```python
from build123d import *
from build123d import SkipClean  # not in build123d's __all__

# Parameters (mm, degrees)
F1_DEPTH = 9
F2_DEPTH = 13
F4_DEPTH = 2.5
F6_DEPTH = 6
F7_R     = 0.5
F8_DEPTH = 10
F9_DEPTH = 2


with BuildPart() as f1:
    # F0 (on Top) → F1 (new body)
    with BuildSketch(Plane.XY):
        with BuildLine():
            ThreePointArc((9.210061901, 13.0833772314), (-14.201425816, -7.3701767138), (16, 0))
            ThreePointArc((16, 0), (15.9921779437, 0.5002445588), (15.9687194227, 1))
            ThreePointArc((15.9687194227, 1), (13.964052369, 7.8105852172), (9.210061901, 13.0833772314))
        make_face()
        with BuildLine():
            Line((10.5963823009, 7.5310478775), (11.473873387, 8.0218594789))
            ThreePointArc((11.473873387, 8.0218594789), (12.2185458229, 6.834262065), (12.8407258, 5.5781503143))
            Line((12.8407258, 5.5781503143), (11.9632347139, 5.0873387129))
            ThreePointArc((11.9632347139, 5.0873387129), (11.1687805133, -6.6526943298), (1.2238876286, -12.9422601995))
            Line((1.2238876286, -12.9422601995), (1.2101974008, -13.9475955724))
            ThreePointArc((1.2101974008, -13.9475955724), (-0.190628347, -13.9987021125), (-1.5895430217, -13.909469903))
            Line((-1.5895430217, -13.909469903), (-1.5758527939, -12.9041345301))
            ThreePointArc((-1.5758527939, -12.9041345301), (-11.3457925498, -6.346100489), (-11.8202699295, 5.4112123221))
            Line((-11.8202699295, 5.4112123221), (-12.6840707878, 5.9257360935))
            ThreePointArc((-12.6840707878, 5.9257360935), (-12.0279174759, 7.1644400474), (-11.2511827783, 8.3313195887))
            Line((-11.2511827783, 8.3313195887), (-10.38738192, 7.8167958172))
            ThreePointArc((-10.38738192, 7.8167958172), (0.1770120365, 12.9987948187), (10.5963823009, 7.5310478775))
        make_face(mode=Mode.SUBTRACT)
        with BuildLine():
            ThreePointArc((9.210061901, 13.0833772314), (13.964052369, 7.8105852172), (15.9687194227, 1))
            Line((15.9687194227, 1), (18.9687194227, 1))
            Line((18.9687194227, 1), (18.9687194227, 16))
            Line((18.9687194227, 16), (12.4687194227, 16))
            Line((12.4687194227, 16), (9.210061901, 13.0833772314))
        make_face()
    extrude(amount=F1_DEPTH)

    # F0 (on Top) → F2 (join)
    with BuildSketch(Plane.XY):
        with BuildLine():
            ThreePointArc((9.210061901, 13.0833772314), (13.964052369, 7.8105852172), (15.9687194227, 1))
            Line((15.9687194227, 1), (18.9687194227, 1))
            Line((18.9687194227, 1), (18.9687194227, 16))
            Line((18.9687194227, 16), (12.4687194227, 16))
            Line((12.4687194227, 16), (9.210061901, 13.0833772314))
        make_face()
    extrude(amount=F2_DEPTH)

    # F3 (on face) → F4 (join)
    with BuildSketch(Plane.YZ.offset(18.9687194227)):
        with BuildLine():
            Line((3.85, 8.35), (3.85, 0))
            Line((3.85, 0), (13.15, 0))
            Line((13.15, 0), (13.15, 8.35))
            ThreePointArc((13.15, 8.35), (11.7880465325, 11.6380465325), (8.5, 13))
            ThreePointArc((8.5, 13), (5.2119534675, 11.6380465325), (3.85, 8.35))
        make_face()
    extrude(amount=F4_DEPTH)

    # F5 (on face) → F6 (join)
    with BuildSketch(Plane.YZ.offset(21.4687194227)):
        with BuildLine():
            Line((0.5, 23), (0.5, 0))
            Line((0.5, 0), (3.85, 0))
            Line((3.85, 0), (3.85, 8.35))
            ThreePointArc((3.85, 8.35), (8.5, 13), (13.15, 8.35))
            Line((13.15, 8.35), (13.15, 0))
            Line((13.15, 0), (16.5, 0))
            Line((16.5, 0), (16.5, 23))
            Line((16.5, 23), (0.5, 23))
        make_face()
        with BuildLine():
            Line((3.85, 8.35), (3.85, 0))
            Line((3.85, 0), (13.15, 0))
            Line((13.15, 0), (13.15, 8.35))
            ThreePointArc((13.15, 8.35), (8.5, 13), (3.85, 8.35))
        make_face()
    extrude(amount=F6_DEPTH)

    # F7 (on face) → F8 (cut)
    with BuildSketch(Plane.YZ.offset(27.4687194227)):
        with Locations((8.5, 7)):
            Circle(F7_R)
        with Locations((8.5, 18)):
            Circle(F7_R)
    extrude(amount=-F8_DEPTH, mode=Mode.SUBTRACT)

    # F0 (on Top) → F9 (join)
    with BuildSketch(Plane.XY):
        with BuildLine():
            ThreePointArc((9.210061901, 13.0833772314), (-14.201425816, -7.3701767138), (16, 0))
            ThreePointArc((16, 0), (15.9921779437, 0.5002445588), (15.9687194227, 1))
            ThreePointArc((15.9687194227, 1), (13.964052369, 7.8105852172), (9.210061901, 13.0833772314))
        make_face()
        with BuildLine():
            Line((10.5963823009, 7.5310478775), (11.473873387, 8.0218594789))
            ThreePointArc((11.473873387, 8.0218594789), (12.2185458229, 6.834262065), (12.8407258, 5.5781503143))
            Line((12.8407258, 5.5781503143), (11.9632347139, 5.0873387129))
            ThreePointArc((11.9632347139, 5.0873387129), (11.1687805133, -6.6526943298), (1.2238876286, -12.9422601995))
            Line((1.2238876286, -12.9422601995), (1.2101974008, -13.9475955724))
            ThreePointArc((1.2101974008, -13.9475955724), (-0.190628347, -13.9987021125), (-1.5895430217, -13.909469903))
            Line((-1.5895430217, -13.909469903), (-1.5758527939, -12.9041345301))
            ThreePointArc((-1.5758527939, -12.9041345301), (-11.3457925498, -6.346100489), (-11.8202699295, 5.4112123221))
            Line((-11.8202699295, 5.4112123221), (-12.6840707878, 5.9257360935))
            ThreePointArc((-12.6840707878, 5.9257360935), (-12.0279174759, 7.1644400474), (-11.2511827783, 8.3313195887))
            Line((-11.2511827783, 8.3313195887), (-10.38738192, 7.8167958172))
            ThreePointArc((-10.38738192, 7.8167958172), (0.1770120365, 12.9987948187), (10.5963823009, 7.5310478775))
        make_face(mode=Mode.SUBTRACT)
    with SkipClean():  # cleaning this boolean's faces spoils the solid; the shape is the same uncleaned
        extrude(amount=-F9_DEPTH)


solid = f1.part
```
Work out the finished part from the listing and answer in its coordinate system (mm). A direction names the side the tool comes from. Give positions to 0.01 mm unless a question says otherwise; leave off trailing zeros. Loops run counter-clockwise (first coordinate to the right, second up) from the corner with the lowest first, then second, coordinate; pieces in that order, holes last. Notation, with made-up numbers: (74, 3) - (94, 3) arc R26 cw to (94, 35) - close; hole circle Ø11 at (83, 23). An arc over 180 degrees is marked (long way). One line per question, with ' | ' between items.
(1) The mould has two halves that part along Y. Classify faces 1 (the face through (27.469, 8, 12)), 2 (the face through (10.86, 14.56, 6.41)), 3 (the face through (23, 9, 7)), 4 (the face through (17.469, 8.5, 7)): +Y half, -Y half, draft (parallel to the pull), parting line (faces both ways), or undercut.
Recorded:
face 1: draft | face 2: +Y half | face 3: undercut | face 4: undercut
(2) The part is cut by section B-B (x = 0). Write down the section's boundary in (y, z).
Recorded:
outline: (-16, -2) - (-14, -2) - (-14, 9) - (-16, 9) - close; (13, -2) - (16, -2) - (16, 9) - (13, 9) - close
(3) A tool of negligible diameter and unlimited length cuts with its end or side. For faces 5 (the face through (20, 3.85, 4)), 6 (the face through (16, 10, 13)), 7 (the face through (18.969, 2, 8)), 8 (the face through (18.969, 15, 6)), 9 (the face through (24, 0.5, 12)), from which of +Z, -Z, +X, -X, +Y, -Y can it reach the whole face along a straight path? Write none if from no direction.
Recorded:
face 5: +Z, -Z, -Y | face 6: +Z, -X, +Y, -Y | face 7: +Z, -Y | face 8: +Z, +Y | face 9: +Z, -Z, +X, -Y
(4) Straight lines are drawn through the part: probe 1 along Z at (x, y) = (25.1, 8.5); probe 2 along Z at (x, y) = (21, 8.5); probe 3 along X at (y, z) = (3, 7.75). For each, find the intervals that lie inside material, in ascending order.
Recorded:
probe 1: z = 0 to 6.5, 7.5 to 17.5, 18.5 to 23 | probe 2: z = 0 to 6.5, 7.5 to 13 | probe 3: x = -15.72 to -12.65, 12.65 to 18.97, 21.47 to 27.47
(5) The part is cut by section D-D (x = 22). Write down the section's boundary in (y, z).
Recorded:
outline: (0.5, 0) - (16.5, 0) - (16.5, 23) - (0.5, 23) - close; hole circle Ø1 at (8.5, 7); hole circle Ø1 at (8.5, 18)
(6) The part is cut by section A-A (z = 18). Write down the section's boundary in (x, y), then the cut area to 3 significant figures.
Recorded:
outline: (21.47, 0.5) - (27.47, 0.5) - (27.47, 8) - (21.47, 8) - close; (21.47, 9) - (27.47, 9) - (27.47, 16.5) - (21.47, 16.5) - close | area: 90.0 mm²
(7) Each of these flat-tipped pins is pushed along its axis until it touches: pin 1 Ø1 at (y, z) = (-2, 6.5) entering from +X; pin 2 Ø3.5 at (x, z) = (14.5, 9.5) entering from +Y; pin 3 Ø5 at (x, z) = (25, 10.5) entering from -Y. Where does it stop, or does it pass through?
Recorded:
pin 1: stops at x = 15.93 | pin 2: stops at y = 16 | pin 3: stops at y = 0.5
